Verification items for the finished model (mm, model axes). Give positions to 0.01 mm unless a question says otherwise; leave off trailing zeros. Order: outer loops, then holes, each group sorted by start corner. A loop starts at its lowest first (then second) coordinate and runs counter-clockwise, first axis right, second up.
(1) Mould release check, pull along X, two halves, no side actions. Record for faces 1 (the face through (-7.493, 0.33, 14.534)), 2 (the face through (0, 0, 12)), 3 (the face through (-0.867, 3.905, 5.916)), 4 (the face through (6, -6, 13.548)): pulls with the +X half, pulls with the -X half, needs draft (parallel to the pull), parting line crosses it, or undercut.
(2) Gauge pin test, flat ends, axial feed: pin 1 (6.5 mm diameter, centred on x = -0.5, y = -1.5, fed in from -Z); pin 2 (5 mm diameter, centred on y = -6.5, z = 15.5, fed in from -X); pin 3 (4 mm diameter, centred on y = 2.5, z = 7, fed in from +X); pin 4 (3 mm diameter, centred on x = 1.5, y = -2.5, fed in from +Z). Record the tip position at first contact, or that the pin passes through.
(3) Scan lines: L1, parallel to Y at x = 0, z = 9; L2, parallel to Z at x = -2.75, y = 9.25; L3, parallel to Y at x = 1.25, z = 5.5. Record each from-to range of solid material in increasing order.
(4) Sectioned sample at A-A on z = 5.25. Record the cut outline in (x, y).
```python
from build123d import *

# Parameters (mm, degrees)
F0_R     = 15
F1_DEPTH = 13.548
F2_R     = 7.5
F3_DEPTH = 2
F5_ANGLE = -180
F6_R     = 4
F7_DEPTH = 12
F8_SIZE  = 1


with BuildPart() as f1:
    # F0 (on Top) → F1 (new body)
    with BuildSketch(Plane.XY):
        Circle(F0_R)
    extrude(amount=F1_DEPTH)

    # F2 (on face) → F3 (join)
    with BuildSketch(Plane.XY.offset(13.548)):
        Circle(F2_R)
    extrude(amount=F3_DEPTH)

    # F4 (on face) → F5 (revolve)
    with BuildSketch(Plane.XY.offset(15.548)):
        with BuildLine():
            Line((0, 7.5), (0, -7.5))
            ThreePointArc((0, -7.5), (5.303301, -5.303301), (7.5, 0))
            ThreePointArc((7.5, 0), (5.303301, 5.303301), (0, 7.5))
        make_face()
    revolve(axis=Axis((0, 0, 15.548), (0, 1, 0)), revolution_arc=F5_ANGLE)

    # F6 (on face) → F7 (cut)
    with BuildSketch(Plane(origin=(0, 0, 0), x_dir=(1, 0, 0), z_dir=(0, 0, -1))):
        Circle(F6_R)
    extrude(amount=-F7_DEPTH, mode=Mode.SUBTRACT)

    # F8
    f8_edges = [f1.edges().sort_by_distance(p)[0] for p in [
        (-15, 0, 13.548),
    ]]
    chamfer(f8_edges, length=F8_SIZE)


solid = f1.part
```
Ans:
1. face 1: parting line crosses it
1. face 2: undercut
1. face 3: undercut
1. face 4: needs draft
2. pin 1: stops at z = 0
2. pin 2: stops at x = -13.25
2. pin 3: stops at x = 14.99
2. pin 4: stops at z = 22.91
3. L1: y = -15 to -4, 4 to 15
3. L2: z = 0 to 13.55
3. L3: y = -14.95 to -3.8, 3.8 to 14.95
4. outline: circle Ø30 at (0, 0); hole circle Ø8 at (0, 0)
